from build123d import *

# Parameters (mm, degrees)
F0_W     = 120
F0_H     = 132
F0_R     = 1.9
F0_R_2   = 4
F1_DEPTH = 5
F2_R     = 4
F3_DEPTH = 25


# Not quite as in the source:
# - a feature names something its author has since deleted; it is built from what else it names


with BuildPart() as f1:
    # F0 (on Top) → F1 (new body)
    with BuildSketch(Plane.XY):
        Rectangle(F0_W, F0_H)
        with Locations((-52, -50)):
            Circle(F0_R, mode=Mode.SUBTRACT)
        with Locations((-20, -50)):
            Circle(F0_R, mode=Mode.SUBTRACT)
        with Locations((-3, -50)):
            Circle(F0_R_2, mode=Mode.SUBTRACT)
        with Locations((12, -50)):
            Circle(F0_R, mode=Mode.SUBTRACT)
        with Locations((44, -50)):
            Circle(F0_R, mode=Mode.SUBTRACT)
    extrude(amount=F1_DEPTH)

    # F2 (on face) → F3 (cut)
    with BuildSketch(Plane.XY.offset(5)):
        with Locations((0, 21)):
            Circle(F2_R)
    extrude(amount=-F3_DEPTH, mode=Mode.SUBTRACT)


solid = f1.part
Geometry check sheet. Reference: the model listing, model coordinates, mm. Give positions to 0.01 mm unless a question says otherwise; leave off trailing zeros. Order: outer loops, then holes, each group sorted by start corner. A loop starts at its lowest first (then second) coordinate and runs counter-clockwise, first axis right, second up.
1) Cross-section at C-C (y = 21). Record the boundary of the cut face in (x, z).
Results are:
outline: (-60, 0) - (-4, 0) - (-4, 5) - (-60, 5) - close; (4, 0) - (60, 0) - (60, 5) - (4, 5) - close
2) Cross-section at A-A (x = -20). Record the boundary of the cut face in (y, z), then the cut area to 3 significant figures.
Results are:
outline: (-66, 0) - (-51.9, 0) - (-51.9, 5) - (-66, 5) - close; (-48.1, 0) - (66, 0) - (66, 5) - (-48.1, 5) - close
area: 641 mm2
3) Draft check along Y on faces 1 (the cylindrical face through (-6.2, -52.4, 2.5)), 2 (the flat face through (-1, -66, 2)), 3 (the flat face through (-1, 1, 5)), 4 (the flat face through (-1, 66, 2)). Enter one of: released by +Y, released by -Y, zero draft, split by the parting line, or undercut.
Results are:
face 1: undercut
face 2: released by -Y
face 3: zero draft
face 4: released by +Y
4) Cross-section at B-B (y = -50). Record the boundary of the cut face in (x, z), then the cut area to 3 significant figures.
Results are:
outline: (-60, 0) - (-53.9, 0) - (-53.9, 5) - (-60, 5) - close; (-50.1, 0) - (-21.9, 0) - (-21.9, 5) - (-50.1, 5) - close; (-18.1, 0) - (-7, 0) - (-7, 5) - (-18.1, 5) - close; (1, 0) - (10.1, 0) - (10.1, 5) - (1, 5) - close; (13.9, 0) - (42.1, 0) - (42.1, 5) - (13.9, 5) - close; (45.9, 0) - (60, 0) - (60, 5) - (45.9, 5) - close
area: 484 mm2
5) Material ranges on probe 1 along Y at (x, z) = (-3, 3.65); probe 2 along X at (y, z) = (21.5, 1.6); probe 3 along Y at (x, z) = (44, 2.65), recorded low to high.
Results are:
probe 1: y = -66 to -54, -46 to 18.35, 23.65 to 66
probe 2: x = -60 to -3.97, 3.97 to 60
probe 3: y = -66 to -51.9, -48.1 to 66
